Part model, mm, in its own coordinate system. A direction names the side the tool comes from. Coordinates: 2 decimals unless noted, no trailing zeros. Order: outer loops, then holes, each group sorted by start corner. A loop starts at its lowest first (then second) coordinate and runs counter-clockwise, first axis right, second up. Notation, with made-up numbers: M -29,4 L 28,4 A23 ccw 28,18 Z; hole C 10.5,83 d6. An arc over 180 degrees is marked long. Write item = value, one per line. Start each with the question number.
Autodesk Inventor part; units mm, degrees
ref_plane "Work Plane2" through (0, 0, 19) normal (0, 0, 1) x (1, 0, 0)
ref_plane "YZ Plane" through (0, 0, 0) normal (1, 0, 0) x (0, 1, 0)
ref_plane "XZ Plane" through (0, 0, 0) normal (0, 1, 0) x (-1, 0, 0)
sketch "Sketch1" plane through (0, 0, 0) normal (1, 0, 0) x (0, 1, 0)
  circle A0 centre (0, 0) radius 16
  circle A1 centre (0, 0) radius 19
  point P0 (19, 0)
  point P1 (0, -19)
  dimension "d0" = 32
  dimension "d1" = 3
extrude "Extrusion1" add sketch "Sketch1" along normal blind 6
ref_plane "Work Plane2" through (0, 0, 19) normal (0, 0, 1) x (1, 0, 0)
sketch "Sketch4" plane through (0, 0, 19) normal (0, 0, 1) x (1, 0, 0)
  line L0 (6, 16) -> (6, -16)
  line L1 (6, 7) -> (-13, 7)
  line L2 (-13, 7) -> (-13, -7)
  line L3 (-13, -7) -> (6, -7)
  line L4 (6, -7) -> (6, 7)
  line L5 (-11, 5) -> (-5, 5)
  line L6 (-5, 5) -> (-5, -5)
  line L7 (-5, -5) -> (-11, -5)
  line L8 (-11, -5) -> (-11, 5)
  point P0 (0, 0)
  point P1 (-13, 0)
  point P2 (-5, 0)
  dimension "d11" = 14
  dimension "d12" = 19
  dimension "d13" = 6
  dimension "d14" = 10
  dimension "d15" = 2
extrude "Extrusion4" add sketch "Sketch4" against normal blind 3
sketch "Sketch5" plane through (0, 0, 16) normal (0, 0, -1) x (-1, 0, 0)
  line L0 (13, 7) -> (13, -7)
  line L1 (13, -7) -> (-6, -7)
  line L2 (13, 7) -> (5, 7)
  line L3 (5, 7) -> (5, -7)
  line L4 (5, -7) -> (13, -7)
  line L5 (13, -7) -> (13, 7)
  line L6 (5, 5) -> (11, 5)
  line L7 (11, 5) -> (11, -5)
  line L8 (11, -5) -> (5, -5)
  point P0 (0, 0)
extrude "Extrusion5" add sketch "Sketch5" along normal blind 6 contours L0 L1 L3 L8 L7 L6 L2
sketch "Sketch6" plane through (-13, 7, 19) normal (0, 1, 0) x (1, 0, 0)
  line L0 (8, 3) -> (8, 9)
  line L1 (8, 7.5) -> (4, 7.5)
  line L2 (4, 7.5) -> (4, 4.5)
  line L3 (4, 4.5) -> (8, 4.5)
  line L4 (8, 4.5) -> (8, 7.5)
  line L5 (2, 0) -> (2, 9)
  line L6 (0, 9) -> (8, 9)
  point P0 (13, 19)
  dimension "d20" = 2
  dimension "d21" = 3
  dimension "d22" = 1.5
extrude "Extrusion6" cut sketch "Sketch6" against normal blind 17.25
ref_plane "Work Plane4" through (0, 0, -19) normal (0, 0, 1) x (1, 0, 0)
sketch "Sketch7" plane through (0, 0, -19) normal (0, 0, 1) x (1, 0, 0)
  circle A0 centre (3, 0) radius 1.5
  circle A1 centre (3, 0) radius 2.5
  line L0 (0, 19) -> (0, -19)
  point P0 (0, 0)
  point P1 (0, 0)
  point P2 (0, 7)
  point P3 (0, -7)
  dimension "d25" = 3
  dimension "d26" = 5
  dimension "d27" = 3
extrude "Extrusion7" add sketch "Sketch7" along normal mid plane 6
sketch "Sketch8" plane through (3, 0, -22) normal (0, 0, -1) x (-1, 0, 0)
  circle A0 centre (0, 0) radius 1.5
  point P0 (3, 0)
extrude "Extrusion8" cut sketch "Sketch8" against normal blind 10.75
properties part number "Dc_Ring"
Item 1: Cut at D-D, the plane x = 3. Write the cut outline in (y, z), and give its area (3 significant figures).
Item 2: Cut at A-A, the plane x = -10.5. Write the cut outline in (y, z), and give its area (3 significant figures).
Item 3: Pull direction X, two halves, no side cores. Call faces 6 (the flat face through (6, -4, 16)), 7 (the flat face through (-3, 0, 16)), 8 (the flat face through (-8, 7, 16)): pulls with the +X half, pulls with the -X half, needs draft (parallel to the pull), parting line crosses it, or undercut.
Item 4: Cut at B-B, the plane z = 0. Write the cut outline in (x, y), and give its area (3 significant figures).
Item 5: Cut at C-C, the plane y = 4.5. Write the cut outline in (x, z), and give its area (3 significant figures).
Item 6: 3-axis set-ups, long thin cutter, end or side, ignore diameter. For faces 1 (the flat face through (-5, 6, 11)), 2 (the flat face through (-8, 5, 16)), 3 (the flat face through (-5, 6, 15)), 4 (the flat face through (-7, -6, 11.5)), 5 (the flat face through (-12, 0, 10)): which of +Z, -Z, +X, -X, +Y, -Y reach the whole face in a straight line?
Item 7: Flat gauge pins, fed straight in: pin 1 (1 mm diameter, centred on y = 6, z = 12.5, fed in from +X); pin 2 (6 mm diameter, centred on y = 7.5, z = -11.5, fed in from -X); pin 3 (3 mm diameter, centred on x = -8.5, z = 16.5, fed in from -Y). Where does each tip first touch, or does it go through?
Item 8: Wall check: line 1 along Y through (x, z) = (3, -20.85); line 2 along X through (y, z) = (0, -18.15); line 3 along X through (y, z) = (-8, -15.5). Give the ranges that are in metal, low to high. Write a range as [from, to].
Filled sheet:
q1.outline = M -7,17.66 A19 ccw -2.5,-18.83 L -2.5,-22 L -1.5,-22 L -1.5,-15.93 A16 cw long 1.5,-15.93 L 1.5,-22 L 2.5,-22 L 2.5,-18.83 A19 ccw 7,17.66 L 7,19 L -7,19 Z
q1.area = 333 mm2
q2.outline = M -7,10 L -5,10 L -5,19 L -7,19 Z; M 5,10 L 7,10 L 7,19 L 5,19 Z
q2.area = 36.0 mm2
q3.face_6 = pulls with the +X half
q3.face_7 = undercut
q3.face_8 = needs draft
q4.outline = M 0,-19 L 6,-19 L 6,-16 L 0,-16 Z; M 0,16 L 6,16 L 6,19 L 0,19 Z
q4.area = 36.0 mm2
q5.outline = M -13,10 L -11,10 L -11,19 L -13,19 Z; M -5,16 L 0,16 L 0,15.35 L 6,15.35 L 6,19 L -5,19 Z; M 0,-18.46 L 6,-18.46 L 6,-15.35 L 0,-15.35 Z
q5.area = 73.5 mm2
q6.face_1 = -Z, +X, +Y, -Y
q6.face_2 = +Z, -Z
q6.face_3 = -Z, +Y, -Y
q6.face_4 = +X, +Y, -Y
q6.face_5 = -Z, +X, -X, +Y, -Y
q7.pin_1 = -9
q7.pin_2 = 0
q7.pin_3 = -7
q8.line_1 = [-2.5, -1.5], [1.5, 2.5]
q8.line_2 = [0, 1.5], [4.5, 6]
q8.line_3 = [0, 6]
